Here's the drawing with two shaded views (mm, measured from the low corner). I have some questions. Give positions to 0.01 mm unless a question says otherwise; leave off trailing zeros. Loops run counter-clockwise (first coordinate to the right, second up) from the corner with the lowest first, then second, coordinate; pieces in that order, holes last. Notation, with made-up numbers: (48, 77.5) -> (81, 77.5) arc R26 cw to (81, 104.5) -> close; hole circle Ø7 at (80, -20.75). An arc over 180 degrees is marked (long way). Write each question's results on one line, items separated by ' | '. Start each with the question number.
Q1. Will these pins go through, and if not, where does the flat tip stop? P1, Ø2, axis at y = 6, z = 26, coming from the -X side; P2, Ø3, axis at y = 6, z = 4, coming from the -X side; P3, Ø12, axis at y = 2.5, z = 24.5, coming from the -X side.
Q2. If I drill on line 1 along Y through (x, z) = (13.5, 30.5) (1 decimal); line 2 along Y through (x, z) = (65, 3); line 3 along X through (y, z) = (8.5, 25), over which ranges is the centre line in solid material (lowest first)?
Q3. If we section it at D-D, the plane y = 19: List the corners of the cut face in (x, z) for me, plus the area to 3 significant figures.
Q4. If we section it at B-B, the plane y = 1.5: List the corners of the cut face in (x, z) for me.
Q5. If we section it at A-A, the plane z = 15: List the corners of the cut face in (x, y) for me, plus the area to 3 significant figures.
Q6. We'd pull the mould along X, two halves only. Please class the marked faces 1, 2, 3 and 4: released by +X, released by -X, zero draft, split by the parting line, or undercut.
Q7. If we section it at C-C, the plane x = 20.32: List the corners of the cut face in (y, z) for me.
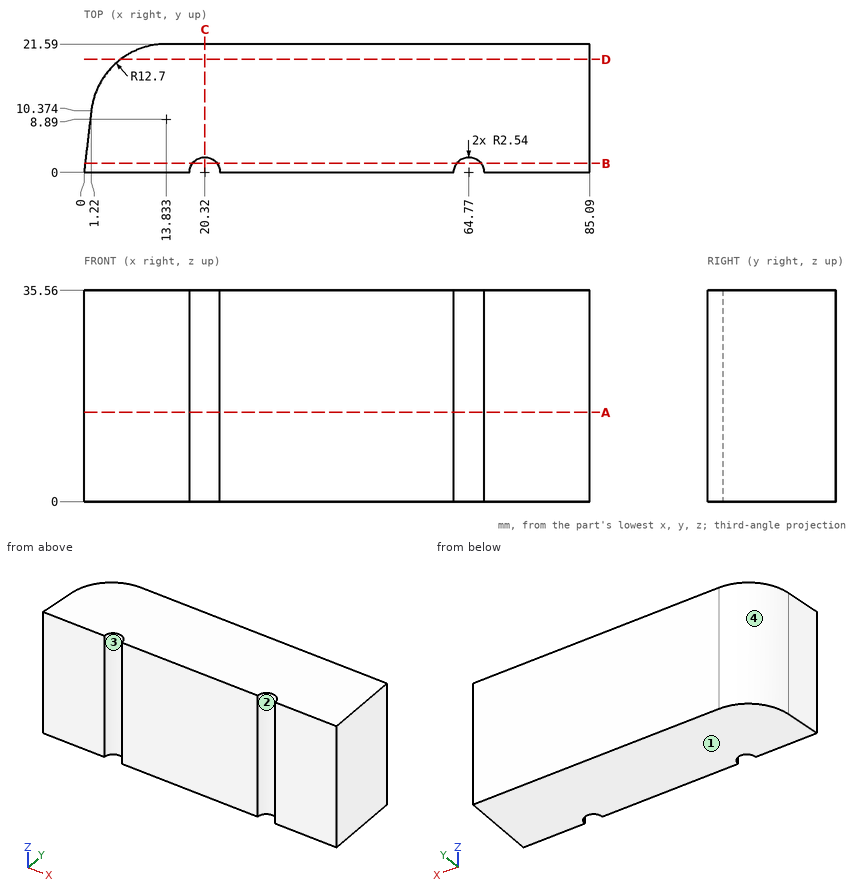
Final values:
1) P1: stops at x = 0.59 | P2: stops at x = 0.53 | P3: stops at x = 0
2) line 1: y = 0 to 21.6 | line 2: y = 2.53 to 21.59 | line 3: x = 1 to 85.09
3) outline: (6.15, 0) -> (85.09, 0) -> (85.09, 35.56) -> (6.15, 35.56) -> close | area: 2,810 mm²
4) outline: (0.18, 0) -> (18.27, 0) -> (18.27, 35.56) -> (0.18, 35.56) -> close; (22.37, 0) -> (62.72, 0) -> (62.72, 35.56) -> (22.37, 35.56) -> close; (66.82, 0) -> (85.09, 0) -> (85.09, 35.56) -> (66.82, 35.56) -> close
5) outline: (0, 0) -> (17.78, 0) arc R2.54 cw to (22.86, 0) -> (62.23, 0) arc R2.54 cw to (67.31, 0) -> (85.09, 0) -> (85.09, 21.59) -> (13.83, 21.59) arc R12.7 ccw to (1.22, 10.37) -> close | area: 1,760 mm²
6) face 1: zero draft | face 2: undercut | face 3: undercut | face 4: released by -X
7) outline: (2.54, 0) -> (21.59, 0) -> (21.59, 35.56) -> (2.54, 35.56) -> close
